Here's how the part is built. I have some questions about the finished solid (model axes, mm). A direction names the side the tool comes from. Give positions to 0.01 mm unless a question says otherwise; leave off trailing zeros. Write each loop counter-clockwise with the first axis right and the second up, starting at its lowest first coordinate (ties: lowest second). Pieces come first, ordered by that corner, then holes. Notation, with made-up numbers: (49, 24.25) -> (80, 24.25) arc R11 cw to (80, 37.25) -> close; hole circle Ø2 at (9, 69). An arc over 180 degrees is marked (long way). Use one line per item in the form item = value.
Autodesk Inventor part; units mm, degrees
ref_plane "YZ Plane" through (0, 0, 0) normal (1, 0, 0) x (0, 1, 0)
ref_plane "XZ Plane" through (0, 0, 0) normal (0, 1, 0) x (-1, 0, 0)
ref_plane "XY Plane" through (0, 0, 0) normal (0, 0, 1) x (1, 0, 0)
sketch "Sketch1" plane through (0, 0, 0) normal (0, 1, 0) x (-1, 0, 0)
  line L0 (32, 55) -> (-32, 55)
  line L1 (-32, 55) -> (-32, -55)
  line L2 (-32, -55) -> (32, -55)
  line L3 (32, -55) -> (32, 55)
  line L4 (32, 55) -> (-32, -55) construction
  line L5 (-32, 55) -> (32, -55) construction
  point P0 (0, 0)
  dimension "d0" = 64
  dimension "d1" = 110
extrude "Extrusion1" add sketch "Sketch1" along normal blind 3
sketch "Sketch2" plane through (0, 3, 0) normal (0, 1, 0) x (1, 0, 0)
  line L0 (-32, -55) -> (32, -55)
  line L1 (32, -55) -> (32, 55)
  line L2 (32, 55) -> (-32, 55)
  line L3 (-32, 55) -> (-32, -55)
  line L4 (-32, -55) -> (32, -55)
  line L5 (32, -55) -> (32, 55)
  line L6 (32, 55) -> (-32, 55)
  line L7 (-32, 55) -> (-32, -55)
  line L8 (-32, -55) -> (32, 55) construction
  line L9 (32, -55) -> (-32, 55) construction
  line L10 (-29, -52) -> (29, -52)
  line L11 (29, -52) -> (29, 52)
  line L12 (29, 52) -> (-29, 52)
  line L13 (-29, 52) -> (-29, -52)
  point P0 (0, 0)
  dimension "d4" = 3
  dimension "d5" = 3
  dimension "d6" = 3
  dimension "d7" = 3
extrude "Extrusion2" add sketch "Sketch2" along normal blind 37
sketch "Sketch3" plane through (0, 3, 0) normal (0, 1, 0) x (1, 0, 0)
  line L0 (-23.08, -46) -> (23.08, -46)
  line L1 (23.08, -46) -> (23.08, 46)
  line L2 (23.08, 46) -> (-23.08, 46)
  line L3 (-23.08, 46) -> (-23.08, -46)
  circle A0 centre (-23.08, -46) radius 1.25
  circle A1 centre (23.08, -46) radius 1.25
  circle A2 centre (23.08, 46) radius 1.25
  circle A3 centre (-23.08, 33) radius 1.25
  line L4 (-29, -52) -> (-29, 52)
  line L5 (29, 52) -> (29, -52)
  line L6 (-29, 52) -> (29, 52)
  line L7 (29, -52) -> (-29, -52)
  circle A4 centre (-23.08, -46) radius 3
  circle A5 centre (-23.08, 33) radius 3
  circle A6 centre (23.08, -46) radius 3
  circle A7 centre (23.08, 46) radius 3
  point P0 (0, 0)
  dimension "d15" = 46.16
  dimension "d16" = 92
  dimension "d17" = 2.5
  dimension "d18" = 2.5
  dimension "d19" = 2.5
  dimension "d20" = 2.5
  dimension "d21" = 79
  dimension "d22" = 5.92
  dimension "d23" = 5.92
  dimension "d24" = 6
  dimension "d25" = 6
  dimension "d26" = 6
  dimension "d27" = 6
  dimension "d28" = 6
  dimension "d29" = 6
extrude "Extrusion3" add sketch "Sketch3" along normal blind 6 contours A0 L3 A4 L0 | L0 A4 L3 A0 | A6 L1 A1 L0 | L0 A1 L1 A6 | A5 L3 A3 | L3 A3 A5 | A7 L2 A2 L1 | L1 A2 L2 A7
sketch "Sketch4" plane through (-29, 3, -52) normal (0, 0, 1) x (1, 0, 0)
  line L0 (8.92, 6) -> (2.92, 6)
  line L1 (5, 4) -> (19, 4)
  line L2 (19, 4) -> (19, 16)
  line L3 (19, 16) -> (5, 16)
  line L4 (5, 16) -> (5, 4)
  line L5 (0, 0) -> (0, 37)
  point P0 (29, -3)
  dimension "d33" = 2
  dimension "d34" = 12
  dimension "d35" = 14
  dimension "d73" = 5
extrude "Extrusion4" cut sketch "Sketch4" against normal blind 6
sketch "Sketch5" plane through (-29, 3, -52) normal (0, 0, 1) x (1, 0, 0)
  line L0 (19, 16) -> (19, 4)
  line L1 (19, 4) -> (5, 4)
  line L2 (5, 4) -> (5, 16)
  line L3 (5, 16) -> (19, 16)
  line L4 (58, 0) -> (0, 0)
  line L5 (58, 0) -> (58, 37)
  line L6 (0, 37) -> (58, 37)
  line L7 (0, 0) -> (0, 37)
  line L8 (23.25, 31) -> (34.75, 31)
  line L9 (34.75, 31) -> (34.75, 24)
  line L10 (34.75, 24) -> (23.25, 24)
  line L11 (23.25, 24) -> (23.25, 31)
  line L12 (8.92, 6) -> (2.92, 6)
  point P0 (29, -3)
  dimension "d38" = 18
  dimension "d39" = 7
  dimension "d40" = 11.5
  dimension "d41" = 23.25
  dimension "d42" = 23.25
extrude "Extrusion5" cut sketch "Sketch5" against normal blind 6 contours L8 L9 L10 L11
sketch "Sketch7" plane through (0, 0, 0) normal (0, -1, 0) x (1, 0, 0)
  line L0 (29, 52) -> (-29, 52)
  line L1 (-29, 52) -> (-29, -52)
  line L2 (-29, -52) -> (29, -52)
  line L3 (29, -52) -> (29, 52)
  line L4 (29, 52) -> (-29, 52)
  line L5 (32, -55) -> (-32, -55)
  line L6 (-32, -55) -> (-32, 55)
  line L7 (-32, 55) -> (32, 55)
  line L8 (32, 55) -> (32, -55)
  line L9 (32, 55) -> (32, -55)
  circle A0 centre (32, 55) radius 4.2426
  point P0 (0, 0)
extrude "Extrusion6" add sketch "Sketch7" against normal blind 40 contours A0 L7 L8 | A0 L8 L7
sketch "Sketch8" plane through (0, 40, 0) normal (0, 1, 0) x (1, 0, 0)
  arc A0 (27.7574, -55) -> (32, -50.7574) centre (32, -55) ccw
  circle A1 centre (32, -55) radius 1.65
  point P0 (0, 0)
  dimension "d47" = 3.3
extrude "Extrusion7" cut sketch "Sketch8" against normal blind 20
mirror "Mirror1" about plane through (0, 0, 0) normal (1, 0, 0) of "Extrusion6", "Extrusion7"
mirror "Mirror2" about plane through (0, 0, 0) normal (0, 0, 1) of "Extrusion6", "Extrusion7", "Mirror1"
sketch "Sketch10" plane through (27.7574, 0, -55) normal (0, 0, -1) x (-1, 0, 0)
  line L0 (21.7574, 0) -> (33.7574, 0)
  line L1 (33.7574, 0) -> (33.7574, 4)
  line L2 (33.7574, 4) -> (21.7574, 4)
  line L3 (21.7574, 4) -> (21.7574, 0)
  line L4 (55.5147, 0) -> (55.5147, 40)
  line L5 (0, 40) -> (0, 0)
  point P0 (27.7574, 0)
  dimension "d56" = 4
  dimension "d57" = 12
  dimension "d58" = 21.7574
  dimension "d59" = 21.7574
extrude "Extrusion9" add sketch "Sketch10" along normal blind 14
chamfer "Chamfer1" distance 2 angle 45 3 edges at (6, 2, -55) (-6, 2, -55) (0, 4, -55)
sketch "Sketch11" plane through (-6, 4, -69) normal (0, 1, 0) x (1, 0, 0)
  line L0 (12, -12) -> (0, -12)
  line L1 (12, -12) -> (12, 0)
  line L2 (0, 0) -> (12, 0)
  line L3 (0, -12) -> (0, 0)
  circle A0 centre (6, -6) radius 2.6
  point P0 (6, -69)
  dimension "d65" = 5.2
  dimension "d66" = 6
  dimension "d67" = 6
extrude "Extrusion10" cut sketch "Sketch11" against normal through all contours A0
mirror "Mirror3" about plane through (0, 0, 0) normal (0, 0, 1) of "Extrusion9", "Extrusion10"
chamfer "Chamfer2" distance 2 angle 45 3 edges at (-6, 2, 55) (0, 4, 55) (6, 2, 55)
equation "\"d4\" = d5"
equation "\"d6\" = d5"
equation "\"d7\" = d5"
equation "\"d22\" = d23"
equation "\"d24\" = d25"
equation "\"d27\" = d26"
equation "\"d28\" = d26"
equation "\"d29\" = d26"
equation "\"d41\" = d42"
equation "\"d58\" = d59"
equation "\"d67\" = d66"
properties part number "Podstawa"
Q1. Will these pins go through, and if not, where does the flat tip stop? pin 1 Ø6 at (x, z) = (-2.5, -65.5) entering from +Y; pin 2 Ø10 at (x, z) = (14.5, -38) entering from +Y; pin 3 Ø1 at (y, z) = (14.5, 47) entering from +X.
Result set:
pin_1 = 4
pin_2 = 3
pin_3 = 32
Q2. I want a section at C-C, the plane x = 0. Write out the boundary of the cut face in (y, z).
Result set:
outline = (0, -69) -> (4, -69) -> (4, -65.6) -> (0, -65.6) -> close; (0, -60.4) -> (4, -60.4) -> (4, -57) -> (6, -55) -> (27, -55) -> (27, -52) -> (3, -52) -> (3, 52) -> (40, 52) -> (40, 55) -> (6, 55) -> (4, 57) -> (4, 60.4) -> (0, 60.4) -> close; (0, 65.6) -> (4, 65.6) -> (4, 69) -> (0, 69) -> close; (34, -55) -> (40, -55) -> (40, -52) -> (34, -52) -> close
Q3. I want a section at A-A, the plane x = -16. Write out the boundary of the cut face in (y, z), and give its area (3 significant figures).
Result set:
outline = (0, -55) -> (7, -55) -> (7, -52) -> (3, -52) -> (3, 52) -> (40, 52) -> (40, 55) -> (0, 55) -> close; (19, -55) -> (40, -55) -> (40, -52) -> (19, -52) -> close
area = 516 mm2
Q4. I want a section at B-B, the plane y = 36. Write out the boundary of the cut face in (x, z), and give its area (3 significant figures).
Result set:
outline = (-32, -50.76) arc R4.24 ccw (long way) to (-27.76, -55) -> (27.76, -55) arc R4.24 ccw (long way) to (32, -50.76) -> (32, 50.76) arc R4.24 ccw (long way) to (27.76, 55) -> (-27.76, 55) arc R4.24 ccw (long way) to (-32, 50.76) -> close; hole circle Ø3.3 at (-32, -55); hole circle Ø3.3 at (-32, 55); hole (-29, -52) -> (29, -52) -> (29, 52) -> (-29, 52) -> close; hole circle Ø3.3 at (32, -55); hole circle Ø3.3 at (32, 55)
area = 1,140 mm2
Q5. If we mould it in two halves opening along X, with no side actions, what happens to faces 6 (the face through (0, 2, 69)), 7 (the face through (29, 21, 1)), 8 (the face through (-22, 9, -32))? For each: +X half, -X half, draft (parallel to the pull), parting line (faces both ways), or undercut.
Result set:
face_6 = draft
face_7 = undercut
face_8 = undercut
Q6. If I drill on line 1 along X through (y, z) = (5, 46); line 2 along X through (y, z) = (4.6, -33); line 3 along Z through (x, y) = (-23, 5), over which ranges is the centre line in solid material (lowest first)? Write a range as from..to.
Result set:
line_1 = -32..-29, -26.08..-24.33, -21.83..-20.08, 20.08..21.83, 24.33..26.08, 29..32
line_2 = -32..-29, -26.08..-24.33, -21.83..-20.08, 29..32
line_3 = -55..-52, -36..-34.25, -31.75..-30, 43..44.75, 47.25..49, 52..55
Q7. I want a section at D-D, the plane z = 31.5. Write out the boundary of the cut face in (x, y), and give its area (3 significant figures).
Result set:
outline = (-32, 0) -> (32, 0) -> (32, 40) -> (29, 40) -> (29, 3) -> (-29, 3) -> (-29, 40) -> (-32, 40) -> close
area = 414 mm2
Q8. Which directions (+Z, -Z, +X, -X, +Y, -Y) give clear straight access to the entire face, cutting with the end or side of a thin tool? Please do faces 1 (the face through (0, 4, 60)), 2 (the face through (-35, 20, 58)), 3 (the face through (0, 4, -60)), 4 (the face through (0, 27, -53)), 5 (the face through (0, 21, 52)).
Result set:
face_1 = +Z, +Y
face_2 = +Y, -Y
face_3 = -Z, +Y
face_4 = -Z
face_5 = +Y
